```python
from build123d import *

# Parameters (mm, degrees)
F0_W     = 84.124804
F0_H     = 114.909604
F1_DEPTH = 12.5
F2_T     = -2.54
F3_R     = 5.08


with BuildPart() as f1:
    # F0 (on Front) → F1 (new body, symmetric)
    with BuildSketch(Plane.XZ):
        Rectangle(F0_W, F0_H)
    extrude(amount=F1_DEPTH, both=True)

    # F2
    f2_openings = [f1.faces().sort_by_distance(p)[0] for p in [
        (0, -12.5, 0),
    ]]
    offset(amount=F2_T, openings=f2_openings)

    # F3
    f3_edges = [f1.edges().sort_by_distance(p)[0] for p in [
        (-42.062402, 0, 57.454802),
        (-42.062402, 0, -57.454802),
        (42.062402, 0, 57.454802),
        (42.062402, 0, -57.454802),
    ]]
    fillet(f3_edges, radius=F3_R)


solid = f1.part
```
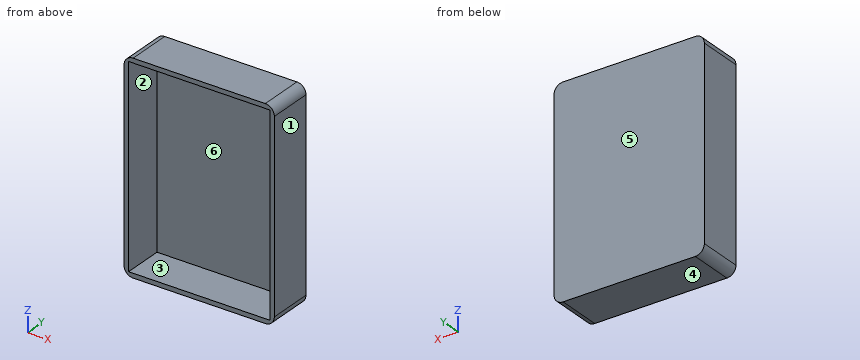
Read the model definition and answer for the solid it produces. Units are mm, in the model's axes. Face numbers are marked on the shaded views. A direction names the side the tool comes from. Coordinates: 2 decimals unless noted, no trailing zeros. Loops run counter-clockwise (first coordinate to the right, second up) from the corner with the lowest first, then second, coordinate; pieces in that order, holes last. Notation, with made-up numbers: (46, 83) -> (76, 83) arc R34 ccw to (76, 122) -> close; hole circle Ø4 at (-34, 74). An arc over 180 degrees is marked (long way). Return JSON: item names as keys, results as strings.
Item 1: Find the intervals of material crossed by probe 1 along X at (y, z) = (-3, 37); probe 2 along Z at (x, y) = (-7, -2.25); probe 3 along Y at (x, z) = (18, 50), in increasing order.
Answers:
{"probe 1": "x = -42.06 to -39.52, 39.52 to 42.06", "probe 2": "z = -57.45 to -54.91, 54.91 to 57.45", "probe 3": "y = 9.96 to 12.5"}
Item 2: Find section A-A (y = 4). Determine the outline of the cut face in (x, z).
Answers:
{"outline": "(-42.06, -52.37) arc R5.08 ccw to (-36.98, -57.45) -> (36.98, -57.45) arc R5.08 ccw to (42.06, -52.37) -> (42.06, 52.37) arc R5.08 ccw to (36.98, 57.45) -> (-36.98, 57.45) arc R5.08 ccw to (-42.06, 52.37) -> close; hole (-39.52, -54.91) -> (39.52, -54.91) -> (39.52, 54.91) -> (-39.52, 54.91) -> close"}
Item 3: Find section C-C (z = -8). Determine the outline of the cut face in (x, y), plus the area to 3 significant figures.
Answers:
{"outline": "(-42.06, -12.5) -> (-39.52, -12.5) -> (-39.52, 9.96) -> (39.52, 9.96) -> (39.52, -12.5) -> (42.06, -12.5) -> (42.06, 12.5) -> (-42.06, 12.5) -> close", "area": "328 mm2"}
Item 4: A flat-ended cylindrical pin translates along its axis: P1, Ø3, axis at x = -2.5, z = 22.5, coming from the -Y side. Find the tip coordinate at first contact, or state that the pin passes through.
Answers:
{"P1": "stops at y = 9.96"}
Item 5: For the marked faces 5 and 6, determine the directions among +Z, -Z, +X, -X, +Y, -Y from which every point of the face is accessible in a straight line to the end or side of a thin tool.
Answers:
{"face 5": "+Z, -Z, +X, -X, +Y", "face 6": "-Y"}
Item 6: Find section B-B (x = -4). Determine the outline of the cut face in (y, z).
Answers:
{"outline": "(-12.5, -57.45) -> (12.5, -57.45) -> (12.5, 57.45) -> (-12.5, 57.45) -> (-12.5, 54.91) -> (9.96, 54.91) -> (9.96, -54.91) -> (-12.5, -54.91) -> close"}
Item 7: For a pull along X with two mould halves and no side action, classify the marked faces 1, 2, 3 and 4 as +X half, -X half, draft (parallel to the pull), parting line (faces both ways), or undercut.
Answers:
{"face 1": "+X half", "face 2": "undercut", "face 3": "undercut", "face 4": "draft"}
